from build123d import *

# Parameters (mm, degrees)
ESQUISSE1_W             = 127.5
ESQUISSE1_H             = 59.5
BOSS_EXTRU_1_DEPTH      = 1
ESQUISSE3_R             = 1.75
ENL_V_MAT_EXTRU_1_DEPTH = 141.703589151
ESQUISSE5_R             = 0.5
ENL_V_MAT_EXTRU_3_DEPTH = 141.703589151
CONG_1_R                = 2


with BuildPart() as part:
    # Esquisse1 → Boss.-Extru.1 (new body)
    with BuildSketch(Plane.XY):
        with Locations((63.75, 29.75)):
            Rectangle(ESQUISSE1_W, ESQUISSE1_H)
    extrude(amount=BOSS_EXTRU_1_DEPTH)

    # Esquisse3 → Enlèv. mat.-Extru.1 (cut, through all)
    with BuildSketch(Plane.XY.offset(1)):
        with Locations((102.85, 6.45)):
            Circle(ESQUISSE3_R)
        with Locations((113.9, 43.75)):
            Circle(ESQUISSE3_R)
        with Locations((23.95, 37.75)):
            Circle(ESQUISSE3_R)
        with Locations((24.65, 6.45)):
            Circle(ESQUISSE3_R)
        Polygon((127.5, 29.5), (121.5, 16.5), (116.7, 16.5), (110.35, 7.5), (106.75, 7.5), (106.75, 0), (127.5, 0), align=None)
        Polygon((0, 0), (20.75, 0), (20.75, 7.5), (17.15, 7.5), (10.8, 16.5), (6, 16.5), (0, 29.5), align=None)
    extrude(amount=-ENL_V_MAT_EXTRU_1_DEPTH, mode=Mode.SUBTRACT)

    # Esquisse5 → Enlèv. mat.-Extru.3 (cut, through all)
    with BuildSketch(Plane.XY.offset(1)):
        with Locations((39.15, 8.5)):
            Circle(ESQUISSE5_R)
        with Locations((88.35, 8.5)):
            Circle(ESQUISSE5_R)
        with Locations((109.25, 19.5)):
            Circle(ESQUISSE5_R)
        with Locations((18.25, 19.5)):
            Circle(ESQUISSE5_R)
    extrude(amount=-ENL_V_MAT_EXTRU_3_DEPTH, mode=Mode.SUBTRACT)

    # Congé1
    cong_1_edges = [part.edges().sort_by_distance(p)[0] for p in [
        (127.5, 29.5, 0.5),
        (106.75, 0, 0.5),
        (110.35, 7.5, 0.5),
        (121.5, 16.5, 0.5),
        (0, 29.5, 0.5),
        (6, 16.5, 0.5),
        (17.15, 7.5, 0.5),
        (20.75, 0, 0.5),
        (0, 59.5, 0.5),
        (127.5, 59.5, 0.5),
    ]]
    fillet(cong_1_edges, radius=CONG_1_R)


solid = part.part
For this review, take the finished solid that the model builds, in its own axes (mm). Give positions to 0.01 mm unless a question says otherwise; leave off trailing zeros. Loops run counter-clockwise (first coordinate to the right, second up) from the corner with the lowest first, then second, coordinate; pieces in that order, holes last.
Item 1: Insertion check: pin 1 (0.5 mm diameter, centred on x = 119, z = 0.5, fed in from -Y); pin 2 (3 mm diameter, centred on x = 113.9, y = 43.75, fed in from -Z); pin 3 (0.5 mm diameter, centred on y = 4, z = 0.5, fed in from -X); pin 4 (0.5 mm diameter, centred on x = 108, z = 0.5, fed in from -Y). Each pin has a flat end and moves straight along its axis. Give the tip position at first contact, or say it passes through.
Item 2: For line 1 along Y through (x, z) = (102.85, 0.8); line 2 along Y through (x, z) = (24.65, 0.55); line 3 along Y through (x, z) = (88.35, 0.2), list the stretches that pass through material, from the lowest coordinate up.
Item 3: Take a section at C-C, the plane z = 0.5. Give the number of separate pieces and of enclosed holes in the cut face, and give its area (3 significant figures).
Item 4: Take a section at A-A, the plane y = 43.75. State the section outline as (x, z) points.
Item 5: Take a section at B-B, the plane x = 102.85. State the section outline as (y, z) points, and give its area (3 significant figures).
Item 6: Take a section at D-D, the plane y = 21.5. State the section outline as (x, z) points.
Item 7: Draft analysis for pull direction Y (two halves, no side actions). For faces 1 (the flat face through (2.86, 23.3, 0.51)), 2 (the cylindrical face through (24.76, 36.2, 0.51)), 3 (the flat face through (63, 30, 1)), state which applies: +Y half, -Y half, draft (parallel to the pull), parting line (faces both ways), or undercut.
Calculated:
1. pin 1: stops at y = 16.5
1. pin 2: passes through
1. pin 3: stops at x = 20.75
1. pin 4: stops at y = 7.5
2. line 1: y = 0 to 4.7, 8.2 to 59.5
2. line 2: y = 0 to 4.7, 8.2 to 36.15, 39.35 to 59.5
2. line 3: y = 0 to 8, 9 to 59.5
3. separate pieces: 1
3. enclosed holes: 8
3. area: 6,900 mm2
4. outline: (0, 0) - (112.15, 0) - (112.15, 1) - (0, 1) - close; (115.65, 0) - (127.5, 0) - (127.5, 1) - (115.65, 1) - close
5. outline: (0, 0) - (4.7, 0) - (4.7, 1) - (0, 1) - close; (8.2, 0) - (59.5, 0) - (59.5, 1) - (8.2, 1) - close
5. area: 56.0 mm2
6. outline: (3.69, 0) - (123.81, 0) - (123.81, 1) - (3.69, 1) - close
7. face 1: -Y half
7. face 2: undercut
7. face 3: draft
